Design review of the part built by this model. Coordinates are the model's own, in mm. Face numbers are marked on the shaded views. A direction names the side the tool comes from. Coordinates: 2 decimals unless noted, no trailing zeros. Loops run counter-clockwise (first coordinate to the right, second up) from the corner with the lowest first, then second, coordinate; pieces in that order, holes last. Notation, with made-up numbers: (-11.75, 10.5) -> (4.25, 10.5) arc R17 cw to (4.25, 25.5) -> close; hole circle Ø2 at (78.5, 69.25). An arc over 180 degrees is marked (long way). One line per item, written item: value. Start each with the question number.
1. Insertion check: pin 1 (1 mm diameter, centred on x = 11, z = 26, fed in from +Y). The pin has a flat end and moves straight along its axis. Give the tip position at first contact, or say it passes through.
2. Machinability: for the marked faces 1 and 2, which of the approach directions +Z, -Z, +X, -X, +Y, -Y give a long, thin tool a straight path to every point of the face, cutting with its end or side? Answer none if there is none.
3. Add section C-C on y = 31.75. Write out the cut boundary in (x, z) (3 decimals), plus the area to 3 significant figures.
4. Add section B-B on z = 57.15. Write out the cut boundary in (x, y) (3 decimals), plus the area to 3 significant figures.
5. For probe 1 along X at (y, z) = (26.5, 25); probe 2 along Y at (x, z) = (13, 40.5); probe 3 along Y at (x, z) = (-1.9, 25.4) (3 decimals), list the stretches that pass through material, from the lowest coordinate up.
6. Draft analysis for pull direction X (two halves, no side actions). For the marked faces 3, 4, 5 and 6, state which applies: pulls with the +X half, pulls with the -X half, needs draft (parallel to the pull), parting line crosses it, or undercut.
7. Add section D-D on z = 46.5. Write out the cut boundary in (x, y), plus the area to 3 significant figures.
8. Add section A-A on y = 16. Write out the cut boundary in (x, z).
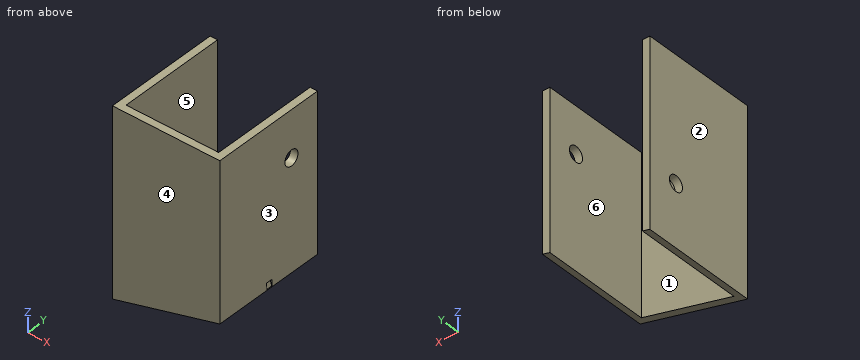
Autodesk Inventor part; units mm, degrees
ref_plane "Work Plane1" through (41.148, 20.701, 11.8423) normal (-0.9659, 0, -0.2588) x (0, 1, 0)
ref_plane "YZ Plane" through (0, 0, 0) normal (1, 0, 0) x (0, 1, 0)
ref_plane "XZ Plane" through (0, 0, 0) normal (0, 1, 0) x (-1, 0, 0)
sketch "Sketch1" plane through (0, 0, 0) normal (0, 0, 1) x (1, 0, 0)
  line L0 (0, 0) -> (38.1, 0)
  line L1 (38.1, 0) -> (38.1, 44.45)
  line L2 (0, 0) -> (0, 44.45)
  line L3 (-3.048, 44.45) -> (-3.048, -3.048)
  line L4 (-3.048, -3.048) -> (41.148, -3.048)
  line L5 (41.148, -3.048) -> (41.148, 44.45)
  line L6 (-3.048, 44.45) -> (0, 44.45)
  line L7 (38.1, 44.45) -> (41.148, 44.45)
  dimension "d0" = 38.1
  dimension "d1" = 44.45
  dimension "d2" = 44.45
  dimension "d3" = 3.048
extrude "channel" add sketch "Sketch1" along normal blind 76.2
sketch "Sketch2" plane through (-3.048, 44.45, 0) normal (0, 1, 0) x (1, 0, 0)
  line L0 (0, 0) -> (49.069, -13.148)
  line L1 (0, 0) -> (50.8, 0) construction
  line L2 (0, 0) -> (49.069, 0)
  line L3 (49.069, -13.148) -> (49.069, 0)
  dimension "d6" = 50.8
  dimension "d7" = 15
extrude "angleCut" cut sketch "Sketch2" against normal blind 101.6
sketch "Sketch3" plane through (41.148, -3.048, 76.2) normal (1, 0, 0) x (0, 0, -1)
  line L0 (64.3577, 47.498) -> (0, 47.498)
  line L1 (0, 0) -> (0, 47.498)
  circle A0 centre (19.05, 34.798) radius 1.7319
  point P0 (76.2, 3.048)
  dimension "d10" = 19.05
  dimension "d11" = 12.7
hole "Hole1" at (41.148, 31.75, 57.15) direction (-1, 0, 0) diameter 6.35 depth 25.4 tip angle 118
sketch "Sketch5" plane through (-3.048, -3.048, 76.2) normal (-1, 0, 0) x (0, 0, 1)
  line L0 (0, 47.498) -> (0, 0)
  line L1 (-76.2, 47.498) -> (0, 47.498)
  circle A0 centre (-50.8, 34.798) radius 3.8194
  point P0 (-76.2, 3.048)
  dimension "d19" = 50.8
  dimension "d20" = 12.7
hole "Hole2" at (-3.048, 31.75, 25.4) direction (1, 0, 0) diameter 6.35 depth 25.4 tip angle 118
ref_plane "Work Plane1" through (41.148, 20.701, 11.8423) normal (-0.9659, 0, -0.2588) x (0, 1, 0)
sketch "Sketch6" plane through (41.148, 20.701, 11.8423) normal (-0.9659, 0, -0.2588) x (0, 1, 0)
  line L0 (1.5352, -0.3226) -> (-1.0048, -0.3226)
  line L1 (-1.0048, -0.3226) -> (-1.0048, -2.8626)
  line L2 (-1.0048, -2.8626) -> (1.5352, -2.8626)
  line L3 (1.5352, -2.8626) -> (1.5352, -0.3226)
  point P0 (-20.701, 0.7889)
  dimension "d29" = 2.54
  dimension "d30" = 2.54
extrude "indentMark" cut sketch "Sketch6" against normal blind 101.6
properties part number "endChannelB" material "Steel, Galvanized"
Worked answers:
1. pin 1: stops at y = 0
2. face 1: +Z, -Z, +Y
2. face 2: +Z, -Z, -X, +Y, -Y
3. outline: (-3.048, 0) -> (0, 0.817) -> (0, 22.225) -> (-3.048, 22.225) -> close; (-3.048, 28.575) -> (0, 28.575) -> (0, 76.2) -> (-3.048, 76.2) -> close; (38.1, 11.026) -> (41.148, 11.842) -> (41.148, 53.975) -> (38.1, 53.975) -> close; (38.1, 60.325) -> (41.148, 60.325) -> (41.148, 76.2) -> (38.1, 76.2) -> close
3. area: 390 mm²
4. outline: (-3.048, -3.048) -> (41.148, -3.048) -> (41.148, 28.575) -> (38.1, 28.575) -> (38.1, 0) -> (0, 0) -> (0, 44.45) -> (-3.048, 44.45) -> close; (38.1, 34.925) -> (41.148, 34.925) -> (41.148, 44.45) -> (38.1, 44.45) -> close
4. area: 386 mm²
5. probe 1: x = -3.05 to 0, 38.1 to 41.15
5. probe 2: y = -3.05 to 0
5. probe 3: y = -3.048 to 28.575, 34.925 to 44.45
6. face 3: pulls with the +X half
6. face 4: needs draft
6. face 5: undercut
6. face 6: undercut
7. outline: (-3.05, -3.05) -> (41.15, -3.05) -> (41.15, 44.45) -> (38.1, 44.45) -> (38.1, 0) -> (0, 0) -> (0, 44.45) -> (-3.05, 44.45) -> close
7. area: 406 mm²
8. outline: (-3.05, 0) -> (0, 0.82) -> (0, 76.2) -> (-3.05, 76.2) -> close; (38.1, 11.03) -> (41.15, 11.84) -> (41.15, 76.2) -> (38.1, 76.2) -> close
